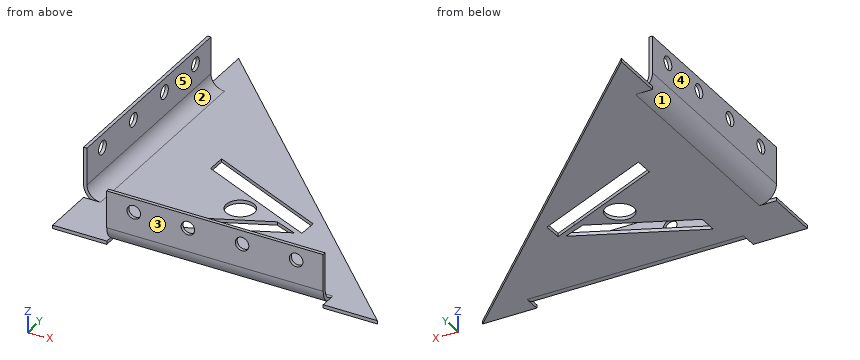
from build123d import *

# Parameters (mm, degrees)
BOSS_EXTRUDE1_DEPTH          = 1.5875
SKETCH7_W                    = 1.5875
SKETCH7_H                    = 101.6
BOSS_EXTRUDE2_DEPTH          = 0.0254
EDGE_FLANGE1_STRIP_W         = 19.05
EDGE_FLANGE1_STRIP_H         = 1.5875
EDGE_FLANGE1_STRIP_CUT_DEPTH = 101.6
EDGE_FLANGE1_DEPTH           = 101.6
SKETCH11_W                   = 101.6
SKETCH11_H                   = 1.5875
BOSS_EXTRUDE3_DEPTH          = 0.0254
EDGE_FLANGE2_STRIP_W         = 19.05
EDGE_FLANGE2_STRIP_H         = 1.5875
EDGE_FLANGE2_STRIP_CUT_DEPTH = 101.6
EDGE_FLANGE2_DEPTH           = 101.6
SKETCH15_R                   = 3.175
CUT_EXTRUDE1_DEPTH           = 2.54
SKETCH16_R                   = 3.175
CUT_EXTRUDE2_DEPTH           = 2.54
SKETCH18_R                   = 6.676012736
CUT_EXTRUDE5_DEPTH           = 2.54


# Sheet-metal steps are written as plain solids
with BuildPart() as part:
    # Sketch1 → Boss-Extrude1 (new body)
    with BuildSketch(Plane.XY):
        Polygon((0, 119.481843199), (0, -32.918156801), (152.4, -32.918156801), align=None)
    extrude(amount=BOSS_EXTRUDE1_DEPTH)

    # Sketch7 → Boss-Extrude2 (add)
    with BuildSketch(Plane.ZY):
        with Locations((0.79375, 43.281843199)):
            Rectangle(SKETCH7_W, SKETCH7_H)
    extrude(amount=BOSS_EXTRUDE2_DEPTH)

    # Edge-Flange1 strip (across the edge) → Edge-Flange1 strip cut (cut)
    with BuildSketch(Plane(origin=(-0.0254, 94.081843199, 1.5875), x_dir=(1, 0, 0), z_dir=(0, -1, 0))):
        with Locations((-1.5875, -0.79375)):
            Rectangle(EDGE_FLANGE1_STRIP_W, EDGE_FLANGE1_STRIP_H)
    extrude(amount=EDGE_FLANGE1_STRIP_CUT_DEPTH, mode=Mode.SUBTRACT)

    # Edge-Flange1 section (across the edge) → Edge-Flange1 (add)
    with BuildSketch(Plane(origin=(-0.0254, 94.081843199, 1.5875), x_dir=(1, 0, 0), z_dir=(0, -1, 0))):
        with BuildLine():
            Line((0, 6.35), (0, 23.8125))
            Line((0, 23.8125), (1.5875, 23.8125))
            Line((1.5875, 23.8125), (1.5875, 6.35))
            ThreePointArc((1.5875, 6.35), (3.447371939, 1.859871939), (7.9375, 0))
            Line((7.9375, 0), (7.9375, -1.5875))
            ThreePointArc((7.9375, -1.5875), (2.324839924, 0.737339924), (0, 6.35))
        make_face()
    extrude(amount=EDGE_FLANGE1_DEPTH)

    # Sketch11 → Boss-Extrude3 (add)
    with BuildSketch(Plane(origin=(0, -32.918156801, 0), x_dir=(-1, 0, 0), z_dir=(0, -1, 0))):
        with Locations((-76.2, -0.79375)):
            Rectangle(SKETCH11_W, SKETCH11_H)
    extrude(amount=BOSS_EXTRUDE3_DEPTH)

    # Edge-Flange2 strip (across the edge) → Edge-Flange2 strip cut (cut)
    with BuildSketch(Plane(origin=(25.4, -32.943556801, 1.5875), x_dir=(0, 1, 0), z_dir=(1, 0, 0))):
        with Locations((-1.5875, -0.79375)):
            Rectangle(EDGE_FLANGE2_STRIP_W, EDGE_FLANGE2_STRIP_H)
    extrude(amount=EDGE_FLANGE2_STRIP_CUT_DEPTH, mode=Mode.SUBTRACT)

    # Edge-Flange2 section (across the edge) → Edge-Flange2 (add)
    with BuildSketch(Plane(origin=(25.4, -32.943556801, 1.5875), x_dir=(0, 1, 0), z_dir=(1, 0, 0))):
        with BuildLine():
            Line((0, 6.35), (0, 23.8125))
            Line((0, 23.8125), (1.5875, 23.8125))
            Line((1.5875, 23.8125), (1.5875, 6.35))
            ThreePointArc((1.5875, 6.35), (3.447371939, 1.859871939), (7.9375, 0))
            Line((7.9375, 0), (7.9375, -1.5875))
            ThreePointArc((7.9375, -1.5875), (2.324839924, 0.737339924), (0, 6.35))
        make_face()
    extrude(amount=EDGE_FLANGE2_DEPTH)

    # Sketch15 → Cut-Extrude1 (cut)
    with BuildSketch(Plane(origin=(0, -31.356056801, 0), x_dir=(1, 0, 0), z_dir=(0, 1, 0))):
        with Locations(Location((38.1, -19.05, 0), (0, 0, 270))):
            Circle(SKETCH15_R)
        with Locations(Location((63.5, -19.05, 0), (0, 0, 270))):
            Circle(SKETCH15_R)
        with Locations(Location((88.9, -19.05, 0), (0, 0, 270))):
            Circle(SKETCH15_R)
        with Locations(Location((114.3, -19.05, 0), (0, 0, 270))):
            Circle(SKETCH15_R)
    extrude(amount=-CUT_EXTRUDE1_DEPTH, mode=Mode.SUBTRACT)

    # Sketch16 → Cut-Extrude2 (cut)
    with BuildSketch(Plane(origin=(1.5621, 0, 0), x_dir=(0, 0, -1), z_dir=(1, 0, 0))):
        with Locations((-19.05, 81.381843199)):
            Circle(SKETCH16_R)
        with Locations((-19.05, 55.981843199)):
            Circle(SKETCH16_R)
        with Locations((-19.05, 30.581843199)):
            Circle(SKETCH16_R)
        with Locations((-19.05, 5.181843199)):
            Circle(SKETCH16_R)
    extrude(amount=-CUT_EXTRUDE2_DEPTH, mode=Mode.SUBTRACT)

    # Sketch18 → Cut-Extrude5 (cut)
    with BuildSketch(Plane(origin=(0, 0, 0), x_dir=(-1, 0, 0), z_dir=(0, 0, -1))):
        with Locations((-59.739888133, 16.534721244)):
            Circle(SKETCH18_R)
        with BuildLine():
            Line((-88.393458916, 10.622584789), (-78.10421078, 14.837125247))
            Line((-78.10421078, 14.837125247), (-33.528048288, -5.335200069))
            add(Edge.make_bspline(
                [(-33.528048288, -5.335200069), (-33.513417888, -8.314924869), (-33.518294688, -11.294649669), (-33.528048288, -14.269497669)],
                knots=[0, 0, 0, 0, 1, 1, 1, 1], degree=3))
            Line((-33.528048288, -14.269497669), (-88.393458916, 10.622584789))
        make_face()
        with BuildLine():
            Line((-91.576598688, 20.702035131), (-91.293744288, 11.938425531))
            Line((-91.293744288, 11.938425531), (-81.408470688, 16.332422331))
            Line((-81.408470688, 16.332422331), (-33.513417888, 38.024428731))
            add(Edge.make_bspline(
                [(-33.532925088, 46.958726331), (-33.503664288, 43.979001531), (-33.532925088, 40.999276731), (-33.513417888, 38.024428731)],
                knots=[0, 0, 0, 0, 1, 1, 1, 1], degree=3))
            Line((-33.532925088, 46.958726331), (-91.576598688, 20.702035131))
        make_face()
    extrude(amount=-CUT_EXTRUDE5_DEPTH, mode=Mode.SUBTRACT)


solid = part.part
The listing builds one solid part. Answer for the finished solid, in the listing's coordinates (mm). Face numbers are marked on the shaded views. A direction names the side the tool comes from. Give positions to 0.01 mm unless a question says otherwise; leave off trailing zeros. Loops run counter-clockwise (first coordinate to the right, second up) from the corner with the lowest first, then second, coordinate; pieces in that order, holes last.
Item 1: Find the intervals of material crossed by line 1 along Y through (x, z) = (0.85, 19.05); line 2 along X through (y, z) = (66.5, 9.75); line 3 along Y through (x, z) = (36, 16.25), in increasing order.
Derived:
line 1: y = -7.52 to 2.01, 8.36 to 27.41, 33.76 to 52.81, 59.16 to 78.21, 84.56 to 94.08
line 2: x = -0.03 to 1.56
line 3: y = -32.94 to -31.36
Item 2: A cutting plane is placed at C-C (x = 38.1). Give the number of separate pieces and of enclosed holes in the cut face, then the cut area to 3 significant figures.
Derived:
separate pieces: 4
enclosed holes: 0
area: 176 mm2
Item 3: A tool of negligible diameter and unlimited length cuts with its end or side. For the marked faces 4 and 5, from which of +Z, -Z, +X, -X, +Y, -Y can it reach the whole face along a straight path? Write none if from no direction.
Derived:
face 4: +Z, -Z, -X, +Y, -Y
face 5: +Z, +X, +Y, -Y
Item 4: A cutting plane is placed at A-A (z = 11.25). Give the vertices of the cut face in (x, y).
Derived:
outline: (-0.03, -7.52) - (1.56, -7.52) - (1.56, 94.08) - (-0.03, 94.08) - close; (25.4, -32.94) - (127, -32.94) - (127, -31.36) - (25.4, -31.36) - close
Item 5: Determine the mould class of the marked faces 1, 2 and 3 for opening direction Y: +Y half, -Y half, draft (parallel to the pull), parting line (faces both ways), or undercut.
Derived:
face 1: undercut
face 2: draft
face 3: -Y half
Item 6: Each of these flat-tipped pins is pushed along its axis until it touches: pin 1 Ø6 at (x, y) = (23.5, 97.5) entering from +Z; pin 2 Ø7.5 at (x, z) = (114.3, 19.05) entering from -Y; pin 3 Ø0.8 at (y, z) = (-29, 0.5) entering from +X; pin 4 Ø8.5 at (y, z) = (-30.5, 14) entering from +X. Where does it stop, or does it pass through?
Derived:
pin 1: stops at z = 1.59
pin 2: stops at y = -32.94
pin 3: stops at x = 148.88
pin 4: stops at x = 127
